Input: part model. Units: mm. Frame: model coordinates. A direction names the side the tool comes from. Coordinates: 2 decimals unless noted, no trailing zeros. Loops run counter-clockwise (first coordinate to the right, second up) from the corner with the lowest first, then second, coordinate; pieces in that order, holes last. Notation, with made-up numbers: (50, 49) - (98, 49) arc R29 ccw to (98, 87) - close; hole circle Ø3 at (44, 22). An arc over 180 degrees is marked (long way). Use a Markdown table: item, result. Add a question column.
1. Section query B-B on y = 0. Return the cut outline in (x, z).
2. Section query D-D on z = 40. Return the cut outline in (x, y).
3. Contact query for flat-ended pins moving along their axis: P1, Ø14, axis at x = -54, y = -3.5, coming from the +Z side; P2, Ø20.5, axis at y = 0, z = 127.02, coming from the -X side; P3, Ø1.5, axis at y = 47.5, z = 96.5, coming from the -X side. Output: stop coordinate, or through.
4. Access query for faces 4 (the face through (-76.469, 45, 15)), 5 (the face through (-48, -1, 29.704)), 6 (the face through (-70, -16.066, 15)). Directions: +Z, -Z, +X, -X, +Y, -Y. A direction counts if a zero-diameter tool reaches every point of the face in a straight line with its end or side. Return the directions, or none.
5. Section query A-A on x = -70. Return the cut outline in (y, z), then the cut area to 3 significant figures.
6. Draft query along Z for faces 1 (the face through (-15, -1, 153.5)), 2 (the face through (-14.64, -1.46, 138.18)), 3 (the face through (0, -1, 76)). Return one class per face: released by +Z, released by -Z, zero draft, split by the parting line, or undercut.
7. Section query C-C on y = -60. Return the cut outline in (x, z), then the cut area to 3 significant figures.
8. Ray query, L1, parallel to Z at x = -12, y = 0; L2, parallel to X at y = 25, z = 47.5; L3, parallel to Z at x = -54, y = 32. Return the intervals inside material, ascending. Write a range as [from, to].
```python
from build123d import *

# Parameters (mm, degrees)
F1_DEPTH = 76.2
F2_R     = 11.250821
F3_DEPTH = 76.469915
F5_DEPTH = 29.704893


with BuildPart() as f1:
    # F0 (on Front) → F1 (new body, symmetric)
    with BuildSketch(Plane.XZ):
        Polygon((-76.468915, 0), (0, 0), (0, 153.50008), (-29.703893, 153.50008), (-29.703893, 29.703893), (-76.468915, 29.703893), align=None)
    extrude(amount=F1_DEPTH, both=True)

    # F2 (on face) → F3 (cut, through all)
    with BuildSketch(Plane.YZ):
        with Locations((0, 127.023965)):
            Circle(F2_R)
    extrude(amount=-F3_DEPTH, mode=Mode.SUBTRACT)

    # F4 (on face) → F5 (cut, through all)
    with BuildSketch(Plane.XY.offset(29.703893)):
        with BuildLine():
            Line((-76.468915, -16.066248), (-63.770004, -16.066248))
            ThreePointArc((-63.770004, -16.066248), (-48.641407, -0.937651), (-63.770004, 14.190945))
            Line((-63.770004, 14.190945), (-76.468915, 14.190945))
            Line((-76.468915, 14.190945), (-76.468915, -16.066248))
        make_face()
    extrude(amount=-F5_DEPTH, mode=Mode.SUBTRACT)


solid = f1.part
```
Resolved:
| question | item | result |
|---|---|---|
| 1 | outline | (-48.67, 0) - (0, 0) - (0, 115.77) - (-29.7, 115.77) - (-29.7, 29.7) - (-48.67, 29.7) - close; (-29.7, 138.27) - (0, 138.27) - (0, 153.5) - (-29.7, 153.5) - close |
| 2 | outline | (-29.7, -76.2) - (0, -76.2) - (0, 76.2) - (-29.7, 76.2) - close |
| 3 | P1 | z = 29.7 |
| 3 | P2 | through |
| 3 | P3 | x = -29.7 |
| 4 | face 4 | +Z, -Z, -X, +Y, -Y |
| 4 | face 5 | +Z, -X, +Y, -Y |
| 4 | face 6 | +Z, -Z, -X |
| 5 | outline | (-76.2, 0) - (-16.07, 0) - (-16.07, 29.7) - (-76.2, 29.7) - close; (14.19, 0) - (76.2, 0) - (76.2, 29.7) - (14.19, 29.7) - close |
| 5 | area | 3,630 mm² |
| 6 | face 1 | released by +Z |
| 6 | face 2 | undercut |
| 6 | face 3 | zero draft |
| 7 | outline | (-76.47, 0) - (0, 0) - (0, 153.5) - (-29.7, 153.5) - (-29.7, 29.7) - (-76.47, 29.7) - close |
| 7 | area | 5,950 mm² |
| 8 | L1 | [0, 115.77], [138.27, 153.5] |
| 8 | L2 | [-29.7, 0] |
| 8 | L3 | [0, 29.7] |
